Geometry check sheet. Reference: the model listing, model coordinates, mm. Face numbers are marked on the shaded views. Coordinates: 2 decimals unless noted, no trailing zeros. Order: outer loops, then holes, each group sorted by start corner. A loop starts at its lowest first (then second) coordinate and runs counter-clockwise, first axis right, second up. Notation, with made-up numbers: (65.25, 30.25) - (100.25, 30.25) arc R28 ccw to (100.25, 64.25) - close; hole circle Ø3 at (-5.75, -2.75). An arc over 180 degrees is marked (long way). Use CSV: the item, a comma, the result in double quotes. Start each with the question number.
1) Sectioned sample at C-C, the plane y = 23.5. Record the cut outline in (x, z).
2) Sectioned sample at B-B, the plane z = -45.5. Record the cut outline in (x, y), and give its area (3 significant figures).
3) Draft check along X on the marked faces 1, 2 and 3. Enter one of: released by +X, released by -X, zero draft, split by the parting line, or undercut.
4) Sectioned sample at A-A, the plane x = 30.5. Record the cut outline in (y, z).
5) Depth check by flat-ended pin: P1, Ø1.5, axis at x = 40, z = -6.5, coming from the +Y side. Enter the tip coordinate at first touch or a pass-through.
6) Thickness scan on probe 1 along Z at (x, y) = (49, 14); probe 2 along X at (y, z) = (29, -15); probe 3 along Y at (x, z) = (28.5, -47). Record the ranges inside material, lowest first. Write a range as [from, to].
7) Sectioned sample at D-D, the plane y = 19.5. Record the cut outline in (x, z), and give its area (3 significant figures).
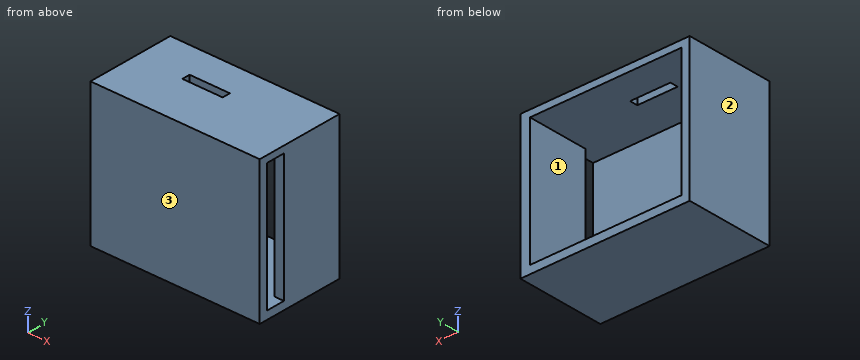
Autodesk Fusion 360 part; units mm, degrees
sketch "Dugnas" plane through (0, 0, 0) normal (0, 1, 0) x (1, 0, 0)
  line L0 (0, 0) -> (63, 0)
  line L1 (63, 0) -> (63, 53)
  line L2 (63, 53) -> (0, 53)
  line L3 (0, 53) -> (0, 0)
  dimension "d1" = 53
  dimension "d2" = 63
extrude "Extrude1" add sketch "Dugnas" along normal blind 3
sketch "Sienos" plane through (0, 3, 0) normal (0, 1, 0) x (-1, 0, 0)
  line L0 (0, -53) -> (0, 0)
  line L1 (0, 0) -> (-63, 0)
  line L2 (-63, 0) -> (-63, -53)
  line L3 (-63, -53) -> (0, -53)
  line L4 (0, 0) -> (-63, -53) construction
  line L5 (0, -53) -> (-63, 0) construction
  line L6 (-3, -2.5238) -> (-59.434, -2.5238)
  line L7 (-59.434, -2.5238) -> (-59.434, -50)
  line L8 (-59.434, -50) -> (-3, -50)
  line L9 (-3, -50) -> (-3, -2.5238)
  dimension "d5" = 3
  dimension "d6" = 3
extrude "Extrude4" add sketch "Sienos" along normal blind 30
sketch "USBC" plane through (59.434, 0, 0) normal (-1, 0, 0) x (0, 0, 1)
  line L0 (-50, 3) -> (-2.5238, 3)
  line L1 (-2.5238, 3) -> (-2.5238, 33)
  line L2 (-2.5238, 33) -> (-50, 33)
  line L3 (-50, 33) -> (-50, 3)
  line L4 (-50, 10) -> (0, 10)
  line L5 (-2.5238, 3) -> (-50, 3)
  dimension "d13" = 7
extrude "Extrude5" cut sketch "USBC" against normal blind 11 contours L0 L1 L3 L4 L5
sketch "LED" plane through (0, 0, -2.5238) normal (0, 0, -1) x (-1, 0, 0)
  line L0 (-63, 3) -> (-3, 3)
  line L1 (-3, 3) -> (-3, 33)
  line L2 (-3, 33) -> (-59.434, 33)
  line L3 (-59.434, 33) -> (-59.434, 10)
  line L4 (-59.434, 10) -> (-63, 10)
  line L5 (-63, 10) -> (-63, 3)
  line L6 (-18, 21) -> (-33, 21)
  line L7 (-33, 21) -> (-33, 18)
  line L8 (-33, 18) -> (-18, 18)
  line L9 (-18, 18) -> (-18, 21)
  line L10 (-3, 3) -> (-59.434, 3)
  point P0 (-63, 3)
  dimension "d16" = 15
  dimension "d17" = 3
  dimension "d18" = 30
  dimension "d19" = 15
extrude "Extrude6" cut sketch "LED" against normal blind 31 contours L6 L7 L8 L9
Evaluation:
1,outline,"(0, -53) - (63, -53) - (63, 0) - (0, 0) - close; hole (3, -50) - (59.43, -50) - (59.43, -2.52) - (3, -2.52) - close"
2,outline,"(0, 0) - (63, 0) - (63, 3) - (3, 3) - (3, 33) - (0, 33) - close; (59.43, 10) - (63, 10) - (63, 33) - (59.43, 33) - close"
2,area,"361 mm²"
3,face 1,"undercut"
3,face 2,"released by -X"
3,face 3,"zero draft"
4,outline,"(0, -53) - (33, -53) - (33, -50) - (3, -50) - (3, -2.52) - (18, -2.52) - (18, 0) - (0, 0) - close; (21, -2.52) - (33, -2.52) - (33, 0) - (21, 0) - close"
5,P1,"y = 3"
6,probe 1,"[-53, -50], [-2.52, 0]"
6,probe 2,"[0, 3], [59.43, 63]"
6,probe 3,"[0, 3]"
7,outline,"(0, -53) - (63, -53) - (63, 0) - (33, 0) - (33, -2.52) - (59.43, -2.52) - (59.43, -50) - (3, -50) - (3, -2.52) - (18, -2.52) - (18, 0) - (0, 0) - close"
7,area,"622 mm²"
